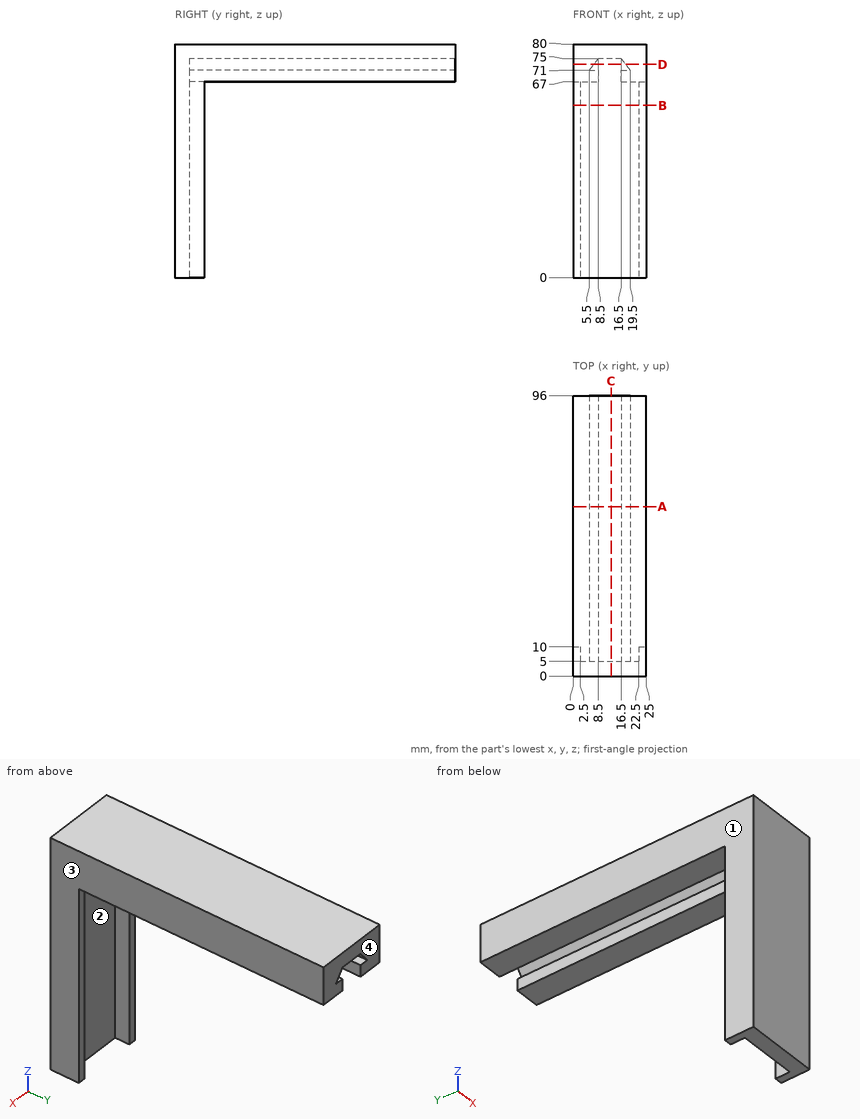
Geometry: see drawing. Coordinates: mm, zero at the bounding-box minimum. Give positions to 0.01 mm unless a question says otherwise; leave off trailing zeros. Loops run counter-clockwise (first coordinate to the right, second up) from the corner with the lowest first, then second, coordinate; pieces in that order, holes last. Notation, with made-up numbers: (13.25, 64.5) -> (47.25, 64.5) arc R22 cw to (47.25, 93.5) -> close; hole circle Ø3 at (-11.75, 34.5). An arc over 180 degrees is marked (long way). Answer as a JSON object with one key per item and string values. Group by question number.
Item 1: Pull-direction query (X, two-part tool) for the marked faces 1, 2, 3 and 4; classes: released by +X, released by -X, zero draft, split by the parting line, or undercut.
Item 2: Cut plane C-C, the plane x = 13. Return the cut outline in (y, z).
Item 3: Cut plane A-A, the plane y = 58. Return the cut outline in (x, z), and give its area (3 significant figures).
Item 4: Cut plane B-B, the plane z = 59. Return the cut outline in (x, y).
Item 5: Cut plane D-D, the plane z = 73. Return the cut outline in (x, y).
Item 6: Line query: probe 1 along Z at (x, y) = (20.5, 22); probe 2 along Y at (x, z) = (17, 17.5); probe 3 along Z at (x, y) = (9, 32). Output: solid intervals per line, ascending.
Item 7: Pin query (flat end, axial travel): P1, Ø6, axis at x = 20.5, y = 26, coming from the -Z side; P2, Ø4, axis at x = 8.5, z = 21, coming from the +Y side; P3, Ø0.8, axis at x = 23.5, z = 32.5, coming from the +Y side. Return the tip coordinate at first contact, or that it passes through.
Checks:
{
 "1": {"face 1": "released by -X", "face 2": "undercut", "face 3": "released by +X", "face 4": "zero draft"},
 "2": {"outline": "(0, 0) -> (5, 0) -> (5, 75) -> (96, 75) -> (96, 80) -> (0, 80) -> close"},
 "3": {"outline": "(0, 67) -> (8.5, 67) -> (8.5, 71) -> (5.5, 71) -> (8.5, 75) -> (16.5, 75) -> (19.5, 71) -> (16.5, 71) -> (16.5, 67) -> (25, 67) -> (25, 80) -> (0, 80) -> close", "area": "249 mm²"},
 "4": {"outline": "(0, 0) -> (25, 0) -> (25, 10) -> (22.5, 10) -> (22.5, 5) -> (2.5, 5) -> (2.5, 10) -> (0, 10) -> close"},
 "5": {"outline": "(0, 0) -> (25, 0) -> (25, 96) -> (18, 96) -> (18, 5) -> (7, 5) -> (7, 96) -> (0, 96) -> close"},
 "6": {"probe 1": "z = 67 to 80", "probe 2": "y = 0 to 5", "probe 3": "z = 75 to 80"},
 "7": {"P1": "stops at z = 67", "P2": "stops at y = 5", "P3": "stops at y = 10"}
}
